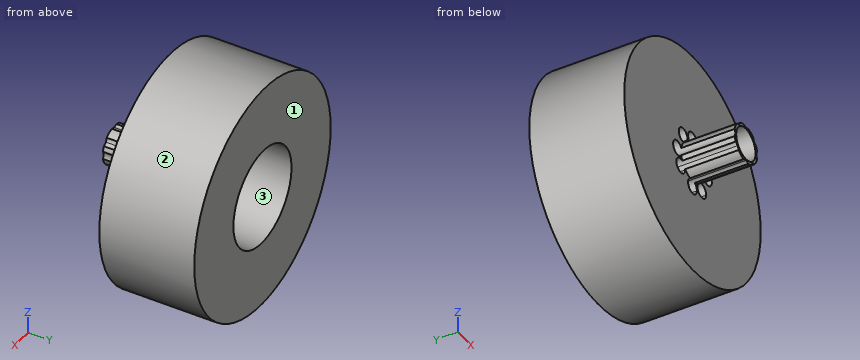
from build123d import *

# Parameters (mm, degrees)
F0_R     = 19.685
F1_DEPTH = 16.256
F2_R     = 8.382
F3_DEPTH = 12.7
F4_R     = 3.302
F5_DEPTH = 9.144
F6_R     = 1.27
F7_DEPTH = 25.4
F8_R     = 2.794
F9_DEPTH = 25.4


# Not quite as in the source:
# - a feature names something its author has since deleted; it is built from what else it names


with BuildPart() as f1:
    # F0 (on Front) → F1 (new body)
    with BuildSketch(Plane.XZ):
        Circle(F0_R)
    extrude(amount=F1_DEPTH)

    # F2 (on Front) → F3 (cut)
    with BuildSketch(Plane.XZ):
        Circle(F2_R)
    extrude(amount=F3_DEPTH, mode=Mode.SUBTRACT)

    # F4 (on face) → F5 (join)
    with BuildSketch(Plane.XZ.offset(16.256)):
        Circle(F4_R)
    extrude(amount=F5_DEPTH)

    # F6 (on Front) → F7 (cut)
    with BuildSketch(Plane.XZ):
        with BuildLine():
            ThreePointArc((1.27, 4.318), (-0.8980256121, 5.2160256121), (0, 3.048))
            ThreePointArc((0, 3.048), (0.8980256121, 3.4199743879), (1.27, 4.318))
        make_face()
        with BuildLine():
            ThreePointArc((-1.4060126705, 3.3888169304), (-3.8189189305, 3.9425906032), (-1.8889501203, 2.3921060685))
            ThreePointArc((-1.8889501203, 2.3921060685), (-1.5331064104, 2.8350432576), (-1.4060126705, 3.3888169304))
        make_face()
        with Locations((-4.318, 0)):
            Circle(F6_R)
        with BuildLine():
            ThreePointArc((-2.1188169304, -2.6760126705), (-2.1890830443, -2.259433023), (-2.3921060685, -1.8889501203))
            ThreePointArc((-2.3921060685, -1.8889501203), (-4.5885508164, -3.092592318), (-2.1188169304, -2.6760126705))
        make_face()
        with BuildLine():
            ThreePointArc((1.27, -4.318), (0.8980256121, -3.4199743879), (0, -3.048))
            ThreePointArc((0, -3.048), (-0.8980256121, -5.2160256121), (1.27, -4.318))
        make_face()
        with BuildLine():
            ThreePointArc((3.9398354632, -3.3809943125), (3.2236091359, -2.2380880524), (1.882772913, -2.3842834506))
            ThreePointArc((1.882772913, -2.3842834506), (2.1160617904, -4.5239005725), (3.9398354632, -3.3809943125))
        make_face()
        with BuildLine():
            ThreePointArc((5.588, 0), (4.318, 1.27), (3.048, 0))
            ThreePointArc((3.048, 0), (4.318, -1.27), (5.588, 0))
        make_face()
        with BuildLine():
            ThreePointArc((4.6588169304, 2.6760126705), (2.9722372829, 3.8757465565), (2.3921060685, 1.8889501203))
            ThreePointArc((2.3921060685, 1.8889501203), (3.8053965779, 1.4762787844), (4.6588169304, 2.6760126705))
        make_face()
    extrude(amount=F7_DEPTH, mode=Mode.SUBTRACT)

    # F8 (on face) → F9 (cut)
    with BuildSketch(Plane(origin=(0, -12.7, 0), x_dir=(-1, 0, 0), z_dir=(0, 1, 0))):
        Circle(F8_R)
    extrude(amount=-F9_DEPTH, mode=Mode.SUBTRACT)


solid = f1.part
Geometry: final body of the model. Coordinates: model frame, mm. Face numbers are marked on the shaded views. Round coordinates to 2 decimals unless told otherwise and drop trailing zeros. Order: outer loops, then holes, each group sorted by start corner. A loop starts at its lowest first (then second) coordinate and runs counter-clockwise, first axis right, second up. Notation, with made-up numbers: (-13, 66.25) - (11, 66.25) arc R27 ccw to (11, 93.25) - close; hole circle Ø3 at (64, -31.75). An arc over 180 degrees is marked (long way). Write each question's results on one line, items separated by ' | '.
Item 1: Section D-D, the plane y = -11.25. Return the cut outline in (x, z) (3 decimals).
Completed:
outline: circle Ø39.37 at (0, 0); hole circle Ø16.764 at (0, 0)
Item 2: Mould query, pull axis X, two halves, no side actions, for the marked faces 1, 2 and 3. Classes: pulls with the +X half, pulls with the -X half, needs draft (parallel to the pull), parting line crosses it, or undercut.
Completed:
face 1: needs draft | face 2: parting line crosses it | face 3: undercut
Item 3: Section A-A, the plane y = -21.75. Return the cut outline in (x, z), and give its area (3 significant figures).
Completed:
outline: (-3.23, -0.66) arc R3.3 ccw to (-2.95, -1.48) arc R1.27 cw to (-2.13, -2.52) arc R3.3 ccw to (-0.66, -3.23) arc R1.27 cw to (0.66, -3.23) arc R3.3 ccw to (1.47, -2.96) arc R1.27 cw to (2.53, -2.12) arc R3.3 ccw to (3.23, -0.66) arc R1.27 cw to (3.23, 0.66) arc R3.3 ccw to (2.95, 1.48) arc R1.27 cw to (2.13, 2.52) arc R3.3 ccw to (0.66, 3.23) arc R1.27 cw to (-0.66, 3.23) arc R3.3 ccw to (-1.48, 2.95) arc R1.27 cw to (-2.52, 2.13) arc R3.3 ccw to (-3.23, 0.66) arc R1.27 cw to start; hole circle Ø5.59 at (0, 0) | area: 7.90 mm^2
Item 4: Section B-B, the plane z = 0. Return the cut outline in (x, y) (3 decimals).
Completed:
outline: (-19.685, -16.256) - (-5.588, -16.256) - (-5.588, -12.7) - (-8.382, -12.7) - (-8.382, 0) - (-19.685, 0) - close; (-3.048, -25.4) - (-2.794, -25.4) - (-2.794, -12.7) - (-3.048, -12.7) - close; (2.794, -25.4) - (3.048, -25.4) - (3.048, -12.7) - (2.794, -12.7) - close; (5.588, -16.256) - (19.685, -16.256) - (19.685, 0) - (8.382, 0) - (8.382, -12.7) - (5.588, -12.7) - close
Item 5: Section C-C, the plane z = -7. Return the cut outline in (x, y).
Completed:
outline: (-18.4, -16.26) - (18.4, -16.26) - (18.4, 0) - (4.61, 0) - (4.61, -12.7) - (-4.61, -12.7) - (-4.61, 0) - (-18.4, 0) - close
Item 6: Material intervals for line 1 along Z through (x, y) = (0, -10) (3 decimals); line 2 along X through (y, z) = (-13, -3); line 3 along Y through (x, z) = (10, 2.5), sorted ascending. Write a range as [from, to].
Completed:
line 1: [-19.685, -8.382], [8.382, 19.685] | line 2: [-19.46, -4.62], [-2.16, 1.46], [3.88, 19.46] | line 3: [-16.26, 0]
Item 7: First-contact query: pin 1 Ø12 at (x, z) = (-14, -5.5) entering from -Y; pin 2 Ø2 at (x, z) = (2.67, -3.38) entering from -Y; pin 3 Ø4 at (x, y) = (0.5, -13) entering from +Z (3 decimals); pin 4 Ø3.5 at (x, z) = (-4.318, 0) entering from +Y. Flat tips, straight axial feed; report the tip coordinate or a pass-through.
Completed:
pin 1: y = -16.26 | pin 2: through | pin 3: z = 19.685 | pin 4: y = -12.7
